from build123d import *

# Parameters (mm, degrees)
CROQUIS1_R                     = 12.7
SALIENTE_EXTRUIR2_DEPTH        = 101.6
TALADRO_ROSCADO_1_2_201_D      = 11.50874
TALADRO_ROSCADO_1_2_201_DEPTH  = 31.75
TALADRO_ROSCADO_1_2_201_TIP    = 3.45757432
TALADRO_ROSCADO_5_16_181_D     = 6.5278
TALADRO_ROSCADO_5_16_181_DEPTH = 19.7485
TALADRO_ROSCADO_5_16_181_TIP   = 1.961148974


with BuildPart() as part:
    # Croquis1 → Saliente-Extruir2 (new, symmetric)
    with BuildSketch(Plane.XY):
        Circle(CROQUIS1_R)
    extrude(amount=SALIENTE_EXTRUIR2_DEPTH, both=True)

    # Taladro roscado 1/2-201
    with Locations(Plane.XY.offset(101.6)):
        with Locations((0, 0)):
            Hole(TALADRO_ROSCADO_1_2_201_D / 2, depth=TALADRO_ROSCADO_1_2_201_DEPTH)
            with Locations((0, 0, -(TALADRO_ROSCADO_1_2_201_DEPTH + TALADRO_ROSCADO_1_2_201_TIP / 2))):  # 118° drill point
                Cone(0, TALADRO_ROSCADO_1_2_201_D / 2, TALADRO_ROSCADO_1_2_201_TIP, mode=Mode.SUBTRACT)

    # Taladro roscado 5/16-181
    with Locations(Plane(origin=(0, 0, -101.6), x_dir=(-1, 0, 0), z_dir=(0, 0, -1))):
        with Locations((0, 0)):
            Hole(TALADRO_ROSCADO_5_16_181_D / 2, depth=TALADRO_ROSCADO_5_16_181_DEPTH)
            with Locations((0, 0, -(TALADRO_ROSCADO_5_16_181_DEPTH + TALADRO_ROSCADO_5_16_181_TIP / 2))):  # 118° drill point
                Cone(0, TALADRO_ROSCADO_5_16_181_D / 2, TALADRO_ROSCADO_5_16_181_TIP, mode=Mode.SUBTRACT)


solid = part.part
Design review of the part built by this model. Coordinates are the model's own, in mm. A direction names the side the tool comes from. Round coordinates to 2 decimals unless told otherwise and drop trailing zeros. Write each loop counter-clockwise with the first axis right and the second up, starting at its lowest first coordinate (ties: lowest second). Pieces come first, ordered by that corner, then holes.
Item 1: Consider section B-B on x = -9.75. Give the boundary of the cut face in (y, z), and give its area (3 significant figures).
Item 2: Wall thickness on L1, parallel to Y at x = 0, z = 84; L2, parallel to X at y = -0.75, z = 22.5: over which ranges is each line inside the solid? List them lowest first.
Item 3: For pin 1 Ø1.5 at (x, z) = (8.5, 68.5) entering from +Y; pin 2 Ø4 at (x, z) = (4, 31.5) entering from -Y; pin 3 Ø1.5 at (y, z) = (-3.5, -81) entering from -X, all flat-tipped, find the tip position at first contact; note any pin that passes through.
Item 4: Draft analysis for pull direction X (two halves, no side actions). For faces 4 (the cylindrical face through (-2.75, -12.4, 1.42)), 5 (the flat face through (3, -3, -101.6)), 6 (the conical face through (0.07, 0.56, -80.23)), state which applies: released by +X, released by -X, zero draft, split by the parting line, or undercut.
Item 5: Consider section C-C on y = -11. Give the boundary of the cut face in (x, z), and give its area (3 significant figures).
Item 6: For faces 1 (the cylindrical face through (-0.708, -3.186, -91.588)), 2 (the flat face through (5.5, -2.6, 101.6)), 3 (the cylindrical face through (0.749, 5.705, 85.503)), list the 3-axis set-ups (+Z, -Z, +X, -X, +Y, -Y) from which the entire face can be reached by the end or side of a thin tool; tool diameter is ignored.
Item 7: Consider section A-A on z = -59. Give the boundary of the cut face in (x, y).
Check values:
1. outline: (-8.14, -101.6) - (8.14, -101.6) - (8.14, 101.6) - (-8.14, 101.6) - close
1. area: 3,310 mm2
2. L1: y = -12.7 to -5.75, 5.75 to 12.7
2. L2: x = -12.68 to 12.68
3. pin 1: stops at y = 10.06
3. pin 2: stops at y = -12.54
3. pin 3: stops at x = -12.4
4. face 4: split by the parting line
4. face 5: zero draft
4. face 6: undercut
5. outline: (-6.35, -101.6) - (6.35, -101.6) - (6.35, 101.6) - (-6.35, 101.6) - close
5. area: 2,580 mm2
6. face 1: -Z
6. face 2: +Z, +X, -X, +Y, -Y
6. face 3: +Z
7. outline: circle Ø25.4 at (0, 0)
